CAD build for the part. Positions are in the model's coordinates, mm. Coordinates: 2 decimals unless noted, no trailing zeros. Order: outer loops, then holes, each group sorted by start corner. A loop starts at its lowest first (then second) coordinate and runs counter-clockwise, first axis right, second up. Notation, with made-up numbers: (47, 14.25) - (65, 14.25) arc R22 cw to (65, 35.25) - close; hole circle Ø5 at (-23.5, 85.5). An arc over 180 degrees is marked (long way). Write each question's results on one line, items separated by ' | '. Start each with the question number.
Q1. Wall check: probe 1 along Z at (x, y) = (-5, 2.8); probe 2 along X at (y, z) = (1.25, -45); probe 3 along Z at (x, y) = (-55, 1.9). Give the ranges that are in metal, low to high.
Q2. Band-saw the part on D-D, the plane x = -5. Write the cut outline in (y, z).
Q3. Band-saw the part on A-A, the plane x = -12.5. Write the cut outline in (y, z).
Q4. Pin check, flat tip, straight feed: P1, Ø1, axis at y = 4.5, z = 28, coming from the +X side. Stop position of the tip, or through.
Q5. Band-saw the part on C-C, the plane y = 1.55. Write the cut outline in (x, z).
Q6. Band-saw the part on B-B, the plane z = 0. Write the cut outline in (x, y).
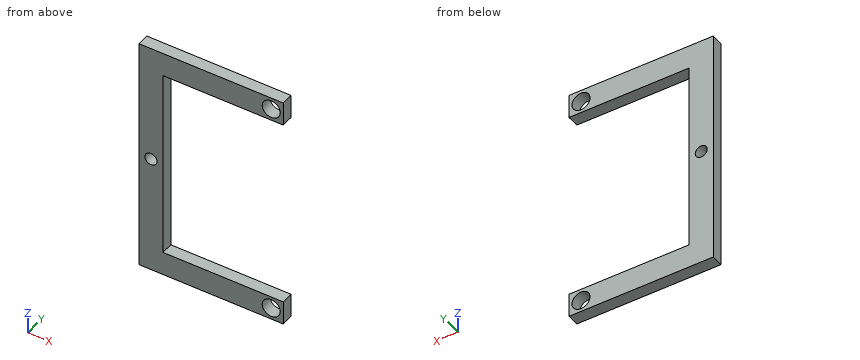
Autodesk Inventor part; units mm, degrees
ref_plane "YZ Plane" through (0, 0, 0) normal (1, 0, 0) x (0, 1, 0)
ref_plane "XZ Plane" through (0, 0, 0) normal (0, 1, 0) x (-1, 0, 0)
ref_plane "XY Plane" through (0, 0, 0) normal (0, 0, 1) x (1, 0, 0)
sketch "スケッチ1" plane through (0, 0, 0) normal (0, 1, 0) x (-1, 0, 0)
  line L0 (72, 0) -> (-12, 0)
  line L1 (0, -70) -> (0, 70)
  line L2 (60, 0) -> (60, -50)
  line L3 (60, -50) -> (0, -50)
  line L4 (0, -40) -> (50, -40)
  line L5 (50, -40) -> (50, 0)
  line L6 (60, 0) -> (60, 50)
  line L7 (60, 50) -> (0, 50)
  line L8 (0, 40) -> (50, 40)
  line L9 (50, 40) -> (50, 0)
  line L10 (0, 50) -> (0, 40)
  line L11 (0, -40) -> (0, -50)
  point P0 (0, 0)
  dimension "d0" = 10
  dimension "d1" = 50
  dimension "d2" = 50
  dimension "d4" = 10
  dimension "d5" = 50
extrude "押し出し1" add sketch "スケッチ1" along normal blind 5 contours L2 L3 L1 L4 L5 L0 | L0 L9 L8 L1 L7 L6
sketch "スケッチ2" plane through (0, 5, 0) normal (0, 1, 0) x (1, 0, 0)
  circle A0 centre (-5, -45) radius 3.75
  line L0 (0, -50) -> (0, -40)
  line L1 (-60, -50) -> (0, -50)
  line L2 (-72, 0) -> (12, 0)
  circle A1 centre (-5, 45) radius 3.75
  circle A2 centre (-55, 0) radius 2.5
  line L3 (-50, -40) -> (-50, 40)
  point P0 (0, 0)
  dimension "d8" = 7.5
  dimension "d9" = 5
  dimension "d10" = 5
  dimension "d11" = 5
  dimension "d12" = 5
extrude "押し出し2" cut sketch "スケッチ2" against normal blind 5
properties part number "bogie" material "アルミニウム 6061"
Results below:
1) probe 1: z = -50 to -48.75, -41.25 to -40, 40 to 41.25, 48.75 to 50 | probe 2: x = -60 to -8.75, -1.25 to 0 | probe 3: z = -50 to -2.5, 2.5 to 50
2) outline: (0, -50) - (5, -50) - (5, -48.75) - (0, -48.75) - close; (0, -41.25) - (5, -41.25) - (5, -40) - (0, -40) - close; (0, 40) - (5, 40) - (5, 41.25) - (0, 41.25) - close; (0, 48.75) - (5, 48.75) - (5, 50) - (0, 50) - close
3) outline: (0, -50) - (5, -50) - (5, -40) - (0, -40) - close; (0, 40) - (5, 40) - (5, 50) - (0, 50) - close
4) P1: stops at x = -50
5) outline: (-60, -50) - (0, -50) - (0, -40) - (-50, -40) - (-50, 40) - (0, 40) - (0, 50) - (-60, 50) - close; hole circle Ø5 at (-55, 0); hole circle Ø7.5 at (-5, -45); hole circle Ø7.5 at (-5, 45)
6) outline: (-60, 0) - (-57.5, 0) - (-57.5, 5) - (-60, 5) - close; (-52.5, 0) - (-50, 0) - (-50, 5) - (-52.5, 5) - close
